```python
from build123d import *

# Parameters (mm, degrees)
F0_W     = 25.4
F0_H     = 50.8
F0_W_2   = 20.32
F0_H_2   = 45.72
F1_DEPTH = 88.9
F2_R     = 14.2875
F3_DEPTH = 50.8
F4_R     = 2.4892
F5_DEPTH = 25.401
F6_R     = 2.4892
F7_DEPTH = 50.801


# Not quite as in the source:
# - a feature names something its author has since deleted; it is built from what else it names


with BuildPart() as f1:
    # F0 (on Top) → F1 (new body)
    with BuildSketch(Plane.XY):
        with Locations((12.7, -25.4)):
            Rectangle(F0_W, F0_H)
        with Locations((12.7, -25.4)):
            Rectangle(F0_W_2, F0_H_2, mode=Mode.SUBTRACT)
    extrude(amount=F1_DEPTH)

    # F2 (on face) → F3 (cut)
    with BuildSketch(Plane.YZ.offset(25.4)):
        with Locations((-25.4, 29.21)):
            Circle(F2_R)
    extrude(amount=-F3_DEPTH, mode=Mode.SUBTRACT)

    # F4 (on face) → F5 (cut, through all)
    with BuildSketch(Plane.YZ.offset(25.4)):
        with Locations((-13.49375, 49.8322299276)):
            Circle(F4_R)
        with Locations((-13.49375, 8.5877700724)):
            Circle(F4_R)
        with Locations((-37.30625, 8.5877700724)):
            Circle(F4_R)
        with Locations((-37.30625, 49.8322299276)):
            Circle(F4_R)
    extrude(amount=-F5_DEPTH, mode=Mode.SUBTRACT)

    # F6 (on face) → F7 (cut, through all)
    with BuildSketch(Plane.XZ.offset(50.8)):
        with Locations((12.7, 12.7)):
            Circle(F6_R)
        with Locations((12.7, 25.4)):
            Circle(F6_R)
        with Locations((12.7, 38.1)):
            Circle(F6_R)
        with Locations((12.7, 50.8)):
            Circle(F6_R)
        with Locations((12.7, 63.5)):
            Circle(F6_R)
        with Locations((12.7, 76.2)):
            Circle(F6_R)
    extrude(amount=-F7_DEPTH, mode=Mode.SUBTRACT)


solid = f1.part
```
Geometry check sheet. Reference: the model listing, model coordinates, mm. A direction names the side the tool comes from. Give positions to 0.01 mm unless a question says otherwise; leave off trailing zeros. Write each loop counter-clockwise with the first axis right and the second up, starting at its lowest first coordinate (ties: lowest second). Pieces come first, ordered by that corner, then holes. Notation, with made-up numbers: (-21, -16) - (11, -16) arc R24 cw to (11, 3) - close; hole circle Ø2 at (40, 9.25). An arc over 180 degrees is marked (long way). Use a Markdown table: item, result.
Q1. Section check C-C, the plane z = 63.5. Enter the section's corners in (x, y), then the cut area to 3 significant figures.
Computed:
| item | result |
|---|---|
| outline | (0, -50.8) - (10.21, -50.8) - (10.21, -48.26) - (2.54, -48.26) - (2.54, -2.54) - (10.21, -2.54) - (10.21, 0) - (0, 0) - close; (15.19, -50.8) - (25.4, -50.8) - (25.4, 0) - (15.19, 0) - (15.19, -2.54) - (22.86, -2.54) - (22.86, -48.26) - (15.19, -48.26) - close |
| area | 336 mm² |
Q2. Section check D-D, the plane z = 50.8. Give the number of separate pieces and of enclosed holes in the cut face, then the cut area to 3 significant figures.
Computed:
| item | result |
|---|---|
| separate pieces | 6 |
| enclosed holes | 0 |
| area | 289 mm² |
Q3. Set-up check for faces 1 (the face through (2.54, -26, 44)), 2 (the face through (1.3, -15.3, 10.3)): record each of +Z, -Z, +X, -X, +Y, -Y from which the full face is reachable in a straight line by a thin tool's end or side.
Computed:
| item | result |
|---|---|
| face 1 | +Z, -Z |
| face 2 | +X, -X |
Q4. Go/stop test with a flat-tipped pin: P1, Ø3, axis at x = 12.7, z = 25.4, coming from the -Y side. Record where the tip stops, or that it passes through.
Computed:
| item | result |
|---|---|
| P1 | passes through |
Q5. Section check A-A, the plane y = -9. Enter the section's corners in (x, z).
Computed:
| item | result |
|---|---|
| outline | (0, 0) - (2.54, 0) - (2.54, 88.9) - (0, 88.9) - close; (22.86, 0) - (25.4, 0) - (25.4, 88.9) - (22.86, 88.9) - close |
Q6. Section check B-B, the plane y = -25.4. Enter the section's corners in (x, z).
Computed:
| item | result |
|---|---|
| outline | (0, 0) - (2.54, 0) - (2.54, 14.92) - (0, 14.92) - close; (0, 43.5) - (2.54, 43.5) - (2.54, 88.9) - (0, 88.9) - close; (22.86, 0) - (25.4, 0) - (25.4, 14.92) - (22.86, 14.92) - close; (22.86, 43.5) - (25.4, 43.5) - (25.4, 88.9) - (22.86, 88.9) - close |
Q7. Thickness scan on L1, parallel to Y at x = 14.75, z = 16; L2, parallel to X at y = -41.5, z = 85; L3, parallel to Z at x = 23.25, y = -26. Record the ranges inside material, lowest first. Write a range as [from, to].
Computed:
| item | result |
|---|---|
| L1 | y = [-50.8, -48.26], [-2.54, 0] |
| L2 | x = [0, 2.54], [22.86, 25.4] |
| L3 | z = [0, 14.94], [43.48, 88.9] |
Q8. Draft check along Y on faces 3 (the face through (1.288, -39.793, 8.697)), 4 (the face through (13, 0, 44)), 5 (the face through (2, -23, 0)). Enter one of: pulls with the +Y half, pulls with the -Y half, needs draft (parallel to the pull), parting line crosses it, or undercut.
Computed:
| item | result |
|---|---|
| face 3 | undercut |
| face 4 | pulls with the +Y half |
| face 5 | needs draft |
